from build123d import *

# Parameters (mm, degrees)
SKETCH1_R           = 2.54
SKETCH1_R_2         = 14.3002
BOSS_EXTRUDE1_DEPTH = 3.175


with BuildPart() as part:
    # Sketch1 → Boss-Extrude1 (new body)
    with BuildSketch(Plane.XY):
        Polygon((-59.693768546, 4.271271353), (-59.693768546, -46.528728647), (128.614138554, -46.528728647), (292.911431822, 117.768564621), (256.990407338, 153.689589105), (107.572089586, 4.271271353), align=None)
        with Locations((141.594566523, -19.421025607)):
            Circle(SKETCH1_R, mode=Mode.SUBTRACT)
        with Locations((150.574822644, -10.440769486)):
            Circle(SKETCH1_R, mode=Mode.SUBTRACT)
        with Locations((159.555078765, -1.460513365)):
            Circle(SKETCH1_R, mode=Mode.SUBTRACT)
        with Locations((168.535334886, 7.519742756)):
            Circle(SKETCH1_R, mode=Mode.SUBTRACT)
        with Locations((177.515591007, 16.499998877)):
            Circle(SKETCH1_R, mode=Mode.SUBTRACT)
        with Locations((186.495847129, 25.480254999)):
            Circle(SKETCH1_R, mode=Mode.SUBTRACT)
        with Locations((195.47610325, 34.46051112)):
            Circle(SKETCH1_R, mode=Mode.SUBTRACT)
        with Locations((204.456359371, 43.440767241)):
            Circle(SKETCH1_R, mode=Mode.SUBTRACT)
        with Locations((213.436615492, 52.421023362)):
            Circle(SKETCH1_R, mode=Mode.SUBTRACT)
        with Locations((222.416871613, 61.401279483)):
            Circle(SKETCH1_R, mode=Mode.SUBTRACT)
        with Locations((231.397127734, 70.381535604)):
            Circle(SKETCH1_R, mode=Mode.SUBTRACT)
        with Locations((240.377383855, 79.361791725)):
            Circle(SKETCH1_R, mode=Mode.SUBTRACT)
        with Locations((11.158871814, -1.812116048)):
            Circle(SKETCH1_R, mode=Mode.SUBTRACT)
        with Locations((24.040159799, -1.812116048)):
            Circle(SKETCH1_R, mode=Mode.SUBTRACT)
        with Locations((36.558871814, -1.812116048)):
            Circle(SKETCH1_R, mode=Mode.SUBTRACT)
        with Locations((49.258871814, -1.812116048)):
            Circle(SKETCH1_R, mode=Mode.SUBTRACT)
        with Locations((61.958871814, -1.812116048)):
            Circle(SKETCH1_R, mode=Mode.SUBTRACT)
        with Locations((87.540159799, -1.812116048)):
            Circle(SKETCH1_R, mode=Mode.SUBTRACT)
        with Locations((100.058871814, -1.812116048)):
            Circle(SKETCH1_R, mode=Mode.SUBTRACT)
        with Locations((112.758871814, -1.812116048)):
            Circle(SKETCH1_R, mode=Mode.SUBTRACT)
        with Locations((112.758871814, -14.512116048)):
            Circle(SKETCH1_R, mode=Mode.SUBTRACT)
        with Locations((112.758871814, -27.212116048)):
            Circle(SKETCH1_R, mode=Mode.SUBTRACT)
        with Locations((112.758871814, -39.912116048)):
            Circle(SKETCH1_R, mode=Mode.SUBTRACT)
        with Locations((100.058871814, -39.912116048)):
            Circle(SKETCH1_R, mode=Mode.SUBTRACT)
        with Locations((87.540159799, -39.912116048)):
            Circle(SKETCH1_R, mode=Mode.SUBTRACT)
        with Locations((61.958871814, -39.912116048)):
            Circle(SKETCH1_R, mode=Mode.SUBTRACT)
        with Locations((49.258871814, -39.912116048)):
            Circle(SKETCH1_R, mode=Mode.SUBTRACT)
        with Locations((24.040159799, -39.912116048)):
            Circle(SKETCH1_R, mode=Mode.SUBTRACT)
        with Locations((11.158871814, -39.912116048)):
            Circle(SKETCH1_R, mode=Mode.SUBTRACT)
        with Locations((-1.541128186, -39.912116048)):
            Circle(SKETCH1_R, mode=Mode.SUBTRACT)
        with Locations((-1.541128186, -27.212116048)):
            Circle(SKETCH1_R, mode=Mode.SUBTRACT)
        with Locations((-1.541128186, -14.512116048)):
            Circle(SKETCH1_R, mode=Mode.SUBTRACT)
        with Locations((-1.541128186, -1.812116048)):
            Circle(SKETCH1_R, mode=Mode.SUBTRACT)
        with Locations((55.2538213, -21.128728647)):
            Circle(SKETCH1_R_2, mode=Mode.SUBTRACT)
        with Locations((-32.8841787, -21.128728647)):
            Circle(SKETCH1_R_2, mode=Mode.SUBTRACT)
        with Locations((257.120708411, 117.898865694)):
            Circle(SKETCH1_R_2, mode=Mode.SUBTRACT)
        with Locations((21.301280743, -21.128728647)):
            Circle(SKETCH1_R_2, mode=Mode.SUBTRACT)
        with Locations((89.0240103, -21.128728647)):
            Circle(SKETCH1_R_2, mode=Mode.SUBTRACT)
        with Locations((156.927029711, 17.705186994)):
            Circle(SKETCH1_R, mode=Mode.SUBTRACT)
        with Locations((165.907285832, 26.685443115)):
            Circle(SKETCH1_R, mode=Mode.SUBTRACT)
        with Locations((174.887541953, 35.665699236)):
            Circle(SKETCH1_R, mode=Mode.SUBTRACT)
        with Locations((183.867798074, 44.645955357)):
            Circle(SKETCH1_R, mode=Mode.SUBTRACT)
        with Locations((192.848054195, 53.626211478)):
            Circle(SKETCH1_R, mode=Mode.SUBTRACT)
        with Locations((201.828310316, 62.606467599)):
            Circle(SKETCH1_R, mode=Mode.SUBTRACT)
        with Locations((210.808566437, 71.58672372)):
            Circle(SKETCH1_R, mode=Mode.SUBTRACT)
        with Locations((219.788822558, 80.566979841)):
            Circle(SKETCH1_R, mode=Mode.SUBTRACT)
    extrude(amount=BOSS_EXTRUDE1_DEPTH)


solid = part.part
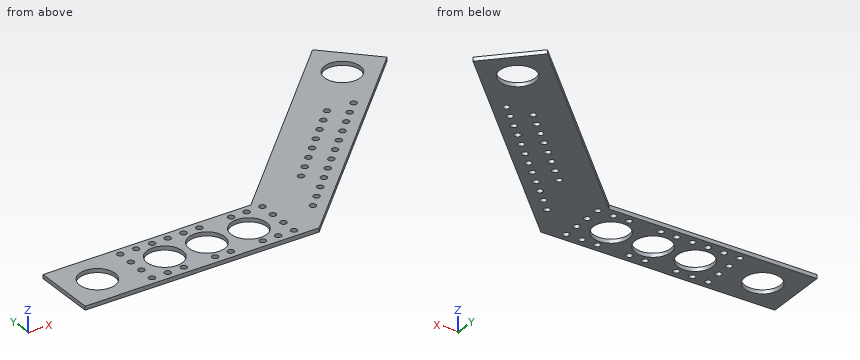
The model under review builds one solid part; all positions refer to its coordinate system, in mm. Round coordinates to 2 decimals unless told otherwise and drop trailing zeros. Order: outer loops, then holes, each group sorted by start corner. A loop starts at its lowest first (then second) coordinate and runs counter-clockwise, first axis right, second up. Notation, with made-up numbers: (-26.5, 68) -> (6.5, 68) arc R21 ccw to (6.5, 82) -> close; hole circle Ø8 at (-3, 59). An arc over 180 degrees is marked (long way). Write item = value, one per line. Start each with the question number.
Item 1: Consider section D-D on y = 135.5. Write out the cut boundary in (x, z) (3 decimals).
Item 2: Consider section C-C on z = 0.55. Count the separate pieces of the cut face and the enclosed holes in it, plus the area to 3 significant figures.
Item 3: Consider section B-B on y = 110.5. Write out the cut boundary in (x, z) (3 decimals).
Item 4: Clearance check with flat-ended pins moving along their axes: pin 1 Ø8 at (x, y) = (87.54, -1.81) entering from +Z (3 decimals); pin 2 Ø1.5 at (y, z) = (78, 0.5) entering from +X. State where each tip first meets the part, or that it passes through.
Item 5: For line 1 along Y through (x, z) = (20, 0.6); line 2 along X through (y, z) = (-19.5, 1.2); line 3 along Y through (x, z) = (151, 0.3), list the stretches that pass through material, from the lowest coordinate up.
Item 6: Consider section A-A on x = 17.5. Write out the cut boundary in (y, z) (3 decimals).
Conclusion:
q1.outline = (238.801, 0) -> (275.18, 0) -> (275.18, 3.175) -> (238.801, 3.175) -> close
q2.separate_pieces = 1
q2.enclosed_holes = 46
q2.area = 16,300 mm2
q3.outline = (213.801, 0) -> (244.883, 0) -> (244.883, 3.175) -> (213.801, 3.175) -> close; (269.358, 0) -> (285.643, 0) -> (285.643, 3.175) -> (269.358, 3.175) -> close
q4.pin_1 = 3.175
q4.pin_2 = 253.89
q5.line_1 = -46.53 to -35.37, -6.89 to 4.27
q5.line_2 = -59.69 to -47.09, -18.68 to 7.09, 35.51 to 41.05, 69.46 to 74.82, 103.23 to 139.06, 144.13 to 155.64
q5.line_3 = -24.14 to -12.94, -7.94 to 47.7
q6.outline = (-46.529, 0) -> (-34.914, 0) -> (-34.914, 3.175) -> (-46.529, 3.175) -> close; (-7.343, 0) -> (4.271, 0) -> (4.271, 3.175) -> (-7.343, 3.175) -> close
